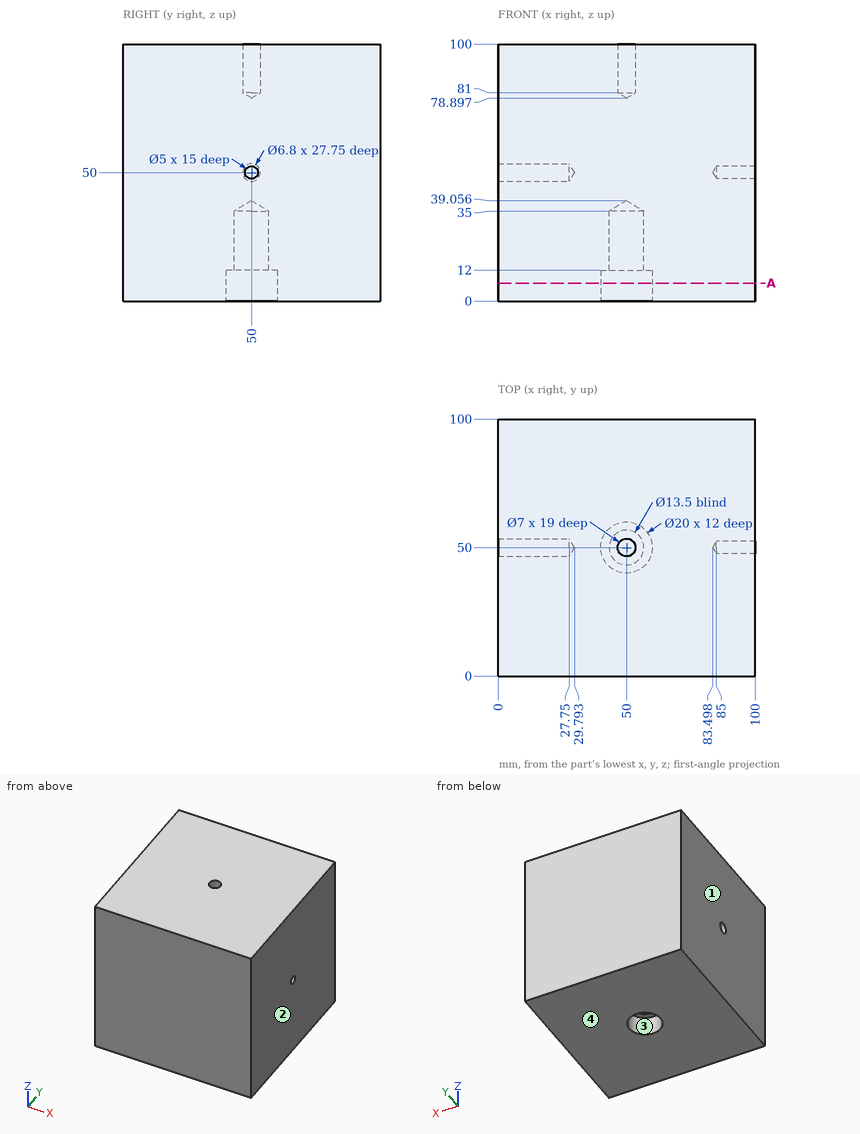
Here's the drawing with two shaded views (mm, measured from the low corner). I have some questions. Give positions to 0.01 mm unless a question says otherwise; leave off trailing zeros. Order: outer loops, then holes, each group sorted by start corner. A loop starts at its lowest first (then second) coordinate and runs counter-clockwise, first axis right, second up. Notation, with made-up numbers: M 5,32 L 25,32 A11 ccw 25,49 Z; hole C -21.75,-10.75 d8. An arc over 180 degrees is marked long. Answer as a JSON object with one key per item and string values. Group by question number.
1) Suppose I cut it at A-A, the plane z = 7. Write out the boundary of the cut face in (x, y).
2) We'd pull the mould along X, two halves only. Please class the marked faces 1, 2, 3 and 4: pulls with the +X half, pulls with the -X half, needs draft (parallel to the pull), parting line crosses it, or undercut.
3) I'm going to push flat-ended pins straight in: pin 1 Ø12 at (x, y) = (50, 50) entering from -Z; pin 2 Ø5.5 at (x, y) = (50, 50) entering from +Z. Where does each tip first touch, or does it pass through?
4) Please list where these lines run through material, in increasing order: L1, parallel to Y at x = 50, z = 86; L2, parallel to Y at x = 93, z = 50. Write a range as [from, to].
Results found:
{
 "1": {"outline": "M 0,0 L 100,0 L 100,100 L 0,100 Z; hole C 50,50 d20"},
 "2": {"face 1": "pulls with the -X half", "face 2": "pulls with the +X half", "face 3": "undercut", "face 4": "needs draft"},
 "3": {"pin 1": "z = 35.45", "pin 2": "z = 80.55"},
 "4": {"L1": "[0, 46.5], [53.5, 100]", "L2": "[0, 47.5], [52.5, 100]"}
}
